```python
from build123d import *

# Parameters (mm, degrees)
F0_R     = 5.4
F0_R_2   = 0.3873329086
F0_R_3   = 3.25
F1_DEPTH = 15


# Not quite as in the source:
# - a fillet or chamfer that OpenCascade refuses, or shapes differently, is made with other operations: its cross-section is extruded or revolved along the edge and cut away or added


with BuildPart() as f1:
    # F0 (on Top) → F1 (new body)
    with BuildSketch(Plane.XY):
        Circle(F0_R)
        with Locations((0, -4.7800762477)):
            Circle(F0_R_2, mode=Mode.SUBTRACT)
        Circle(F0_R_3, mode=Mode.SUBTRACT)
    extrude(amount=F1_DEPTH)

    # F2: chamfer of 0.25 on 3 edges, made by hand

    # F2_s1 → F2_t2 (revolve, cut)
    with BuildSketch(Plane.XZ):
        Polygon((3.25, 14.75), (3.5, 15), (3.25, 15), align=None)
    revolve(axis=Axis((0, 0, 15), (0, 0, 1)), mode=Mode.SUBTRACT)

    # F2_s3 → F2_t4 (revolve, cut)
    with BuildSketch(Plane.XZ):
        Polygon((5.4, 14.75), (5.15, 15), (5.4, 15), align=None)
    revolve(axis=Axis((0, 0, 15), (0, 0, 1)), mode=Mode.SUBTRACT)

    # F2_s5 → F2_t6 (revolve, cut)
    with BuildSketch(Plane.XZ):
        Polygon((3.25, 0.25), (3.5, 0), (3.25, 0), align=None)
    revolve(axis=Axis((0, 0, 0), (0, 0, 1)), mode=Mode.SUBTRACT)

    # F3: chamfer of 0.25 on 1 edges, made by hand

    # F3_s1 → F3_t2 (revolve, cut)
    with BuildSketch(Plane.XZ):
        Polygon((5.4, 0.25), (5.15, 0), (5.4, 0), align=None)
    revolve(axis=Axis((0, 0, 0), (0, 0, 1)), mode=Mode.SUBTRACT)


solid = f1.part
```
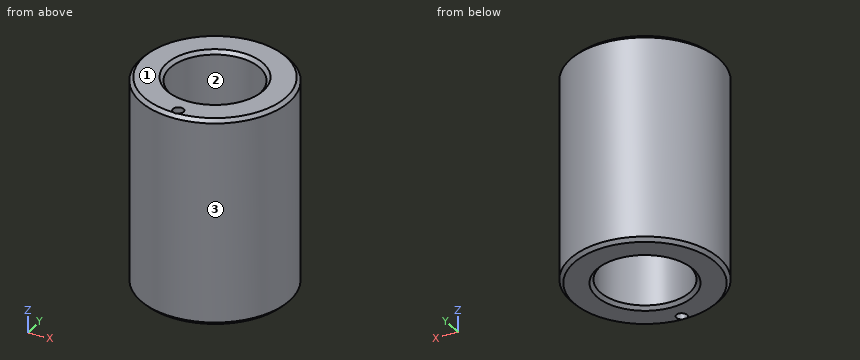
CAD build for the part. Positions are in the model's coordinates, mm. Face numbers are marked on the shaded views. Coordinates: 2 decimals unless noted, no trailing zeros. Write each loop counter-clockwise with the first axis right and the second up, starting at its lowest first coordinate (ties: lowest second). Pieces come first, ordered by that corner, then holes. Notation, with made-up numbers: (3, 26) -> (23, 26) arc R24 ccw to (23, 44) -> close; hole circle Ø9 at (68, 26.25). An arc over 180 degrees is marked (long way). Use CSV: the item, a comma, the result in double quotes. Start each with the question number.
Item 1: Two-plate mould, pull along X, no slides. Class the marked faces 1, 2 and 3: +X half, -X half, draft (parallel to the pull), parting line (faces both ways), or undercut.
Item 2: Band-saw the part on A-A, the plane y = 0. Write the cut outline in (x, z).
Item 3: Wall check: probe 1 along Y at (x, z) = (0, 6); probe 2 along X at (y, z) = (1, 2.5); probe 3 along Y at (x, z) = (-0.5, 8.5). Give the ranges that are in metal, low to high.
Item 4: Drop flat-ended pins along their axis: P1, Ø1.5, axis at x = 2, y = 1, coming from the -Z side; P2, Ø1, axis at y = 3, z = 8.5, coming from the -X side. Give the stop position or say it passes through.
Item 5: Band-saw the part on B-B, the plane z = 8.75. Write the cut outline in (x, y).
Response values:
1,face 1,"draft"
1,face 2,"undercut"
1,face 3,"parting line"
2,outline,"(-5.4, 0.25) -> (-5.15, 0) -> (-3.5, 0) -> (-3.25, 0.25) -> (-3.25, 14.75) -> (-3.5, 15) -> (-5.15, 15) -> (-5.4, 14.75) -> close; (3.25, 0.25) -> (3.5, 0) -> (5.15, 0) -> (5.4, 0.25) -> (5.4, 14.75) -> (5.15, 15) -> (3.5, 15) -> (3.25, 14.75) -> close"
3,probe 1,"y = -5.4 to -5.17, -4.39 to -3.25, 3.25 to 5.4"
3,probe 2,"x = -5.31 to -3.09, 3.09 to 5.31"
3,probe 3,"y = -5.38 to -3.21, 3.21 to 5.38"
4,P1,"passes through"
4,P2,"stops at x = -4.79"
5,outline,"circle Ø10.8 at (0, 0); hole circle Ø6.5 at (0, 0); hole circle Ø0.77 at (0, -4.78)"
